Print and shaded views of the part. All mm, measured from the part's lowest x, y and z. A direction names the side the tool comes from. Round coordinates to 2 decimals unless told otherwise and drop trailing zeros. Loops run counter-clockwise (first coordinate to the right, second up) from the corner with the lowest first, then second, coordinate; pieces in that order, holes last. Notation, with made-up numbers: (-15.5, 34.5) -> (8.5, 34.5) arc R27 ccw to (8.5, 61.5) -> close; hole circle Ø5 at (-10, 25). An arc over 180 degrees is marked (long way). Answer as CSV lines item,"result".
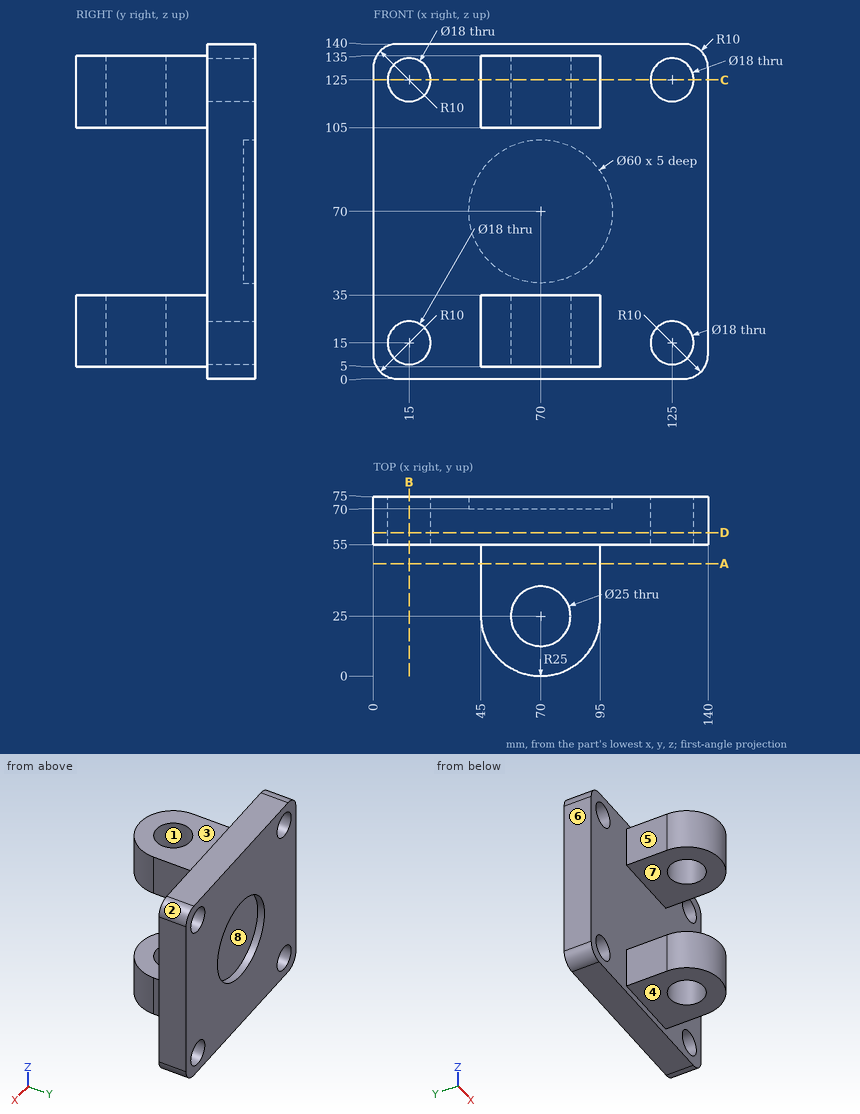
Q1. Saw through at B-B, the plane x = 15. Write the cut outline in (y, z), then the cut area to 3 significant figures.
Geometry results:
outline,"(55, 0) -> (75, 0) -> (75, 6) -> (55, 6) -> close; (55, 24) -> (75, 24) -> (75, 116) -> (55, 116) -> close; (55, 134) -> (75, 134) -> (75, 140) -> (55, 140) -> close"
area,"2,080 mm2"
Q2. Two-plate mould, pull along X, no slides. Class the marked faces 1, 2 and 3: pulls with the +X half, pulls with the -X half, needs draft (parallel to the pull), parting line crosses it, or undercut.
Geometry results:
face 1,"undercut"
face 2,"pulls with the +X half"
face 3,"needs draft"
Q3. Saw through at D-D, the plane y = 60. Write the cut outline in (x, z).
Geometry results:
outline,"(0, 10) arc R10 ccw to (10, 0) -> (130, 0) arc R10 ccw to (140, 10) -> (140, 130) arc R10 ccw to (130, 140) -> (10, 140) arc R10 ccw to (0, 130) -> close; hole circle Ø18 at (15, 15); hole circle Ø18 at (15, 125); hole circle Ø18 at (125, 15); hole circle Ø18 at (125, 125)"
Q4. Saw through at A-A, the plane y = 47. Write the cut outline in (x, z).
Geometry results:
outline,"(45, 5) -> (95, 5) -> (95, 35) -> (45, 35) -> close; (45, 105) -> (95, 105) -> (95, 135) -> (45, 135) -> close"
Q5. Saw through at C-C, the plane z = 125. Write the cut outline in (x, y).
Geometry results:
outline,"(0, 55) -> (6, 55) -> (6, 75) -> (0, 75) -> close; (24, 55) -> (45, 55) -> (45, 25) arc R25 ccw to (95, 25) -> (95, 55) -> (116, 55) -> (116, 75) -> (24, 75) -> close; (134, 55) -> (140, 55) -> (140, 75) -> (134, 75) -> close; hole circle Ø25 at (70, 25)"
Q6. Drop flat-ended pins along their axis: P1, Ø3, axis at x = 94.5, y = 23.5, coming from the +Z side; P2, Ø8, axis at y = 34.5, z = 99.5, coming from the -X side; P3, Ø23.5, axis at x = 15, z = 15, coming from the -Y side; P4, Ø9, axis at y = 44.5, z = 114.5, coming from the +X side. Give the stop position or say it passes through.
Geometry results:
P1,"z = 135"
P2,"through"
P3,"y = 55"
P4,"x = 95"
Q7. Drill centre lines: line 1 along Z through (x, y) = (125, 69.25); line 2 along Y through (x, z) = (70, 122); line 3 along Z through (x, y) = (66.5, 37.5). Where is each one in solid material? Low to high.
Geometry results:
line 1,"0 to 6, 24 to 116, 134 to 140"
line 2,"0 to 12.5, 37.5 to 75"
line 3,"5 to 35, 105 to 135"
Q8. Which spindle directions (+Z, -Z, +X, -X, +Y, -Y) get a long thin tool onto all of the face, cutting with end or side? Do the marked faces 4, 5, 6, 7 and 8. Say none if no direction does.
Geometry results:
face 4,"-Z, +X, -X, -Y"
face 5,"+Z, -Z, -X, -Y"
face 6,"+Z, -Z, -X, +Y, -Y"
face 7,"+X, -X, -Y"
face 8,"+Y"
